```python
from build123d import *

# Parameters (mm, degrees)
BOSS_EXTRUDE1_START     = -21.43125
SKETCH4_R               = 6.35
BOSS_EXTRUDE1_DEPTH     = 42.8625
SKETCH5_R               = 1.984375
CUT_EXTRUDE1_DEPTH      = 42.828441001
CHAMFER1_SIZE           = 0.6985
CUT_EXTRUDE3_REACH      = 52.483
CUT_EXTRUDE3_END_RADIUS = 6.35
SKETCH7_R               = 2.4257


with BuildPart() as part:
    # Sketch4 → Boss-Extrude1 (new body)
    with BuildSketch(Plane.XY.offset(BOSS_EXTRUDE1_START)):
        with BuildLine():
            Line((-25.4, -9.525), (-17.4625, -9.525))
            Line((-17.4625, -9.525), (-17.4625, 12.7))
            Line((-17.4625, 12.7), (-10.4775, 12.7))
            ThreePointArc((-10.4775, 12.7), (0, 15.875), (10.4775, 12.7))
            Line((10.4775, 12.7), (17.4625, 12.7))
            Line((17.4625, 12.7), (17.4625, -9.525))
            Line((17.4625, -9.525), (25.4, -9.525))
            Line((25.4, -9.525), (25.4, -15.875))
            Line((25.4, -15.875), (9.42975, -15.875))
            Line((9.42975, -15.875), (9.42975, -15.5575))
            Line((9.42975, -15.5575), (-9.42975, -15.5575))
            Line((-9.42975, -15.5575), (-9.42975, -15.875))
            Line((-9.42975, -15.875), (-25.4, -15.875))
            Line((-25.4, -15.875), (-25.4, -9.525))
        make_face()
        with Locations((0, 1.5748)):
            Circle(SKETCH4_R, mode=Mode.SUBTRACT)
    extrude(amount=BOSS_EXTRUDE1_DEPTH)

    # Sketch5 → Cut-Extrude1 (cut, through all)
    with BuildSketch(Plane(origin=(0, -9.525, 0), x_dir=(1, 0, 0), z_dir=(0, 1, 0))):
        with Locations(Location((-21.4376, 12.7, 0), (0, 0, 180))):
            Circle(SKETCH5_R)
        with Locations(Location((21.4376, 12.7, 0), (0, 0, 180))):
            Circle(SKETCH5_R)
        with Locations(Location((21.4376, -12.7, 0), (0, 0, 180))):
            Circle(SKETCH5_R)
        with Locations(Location((-21.4376, -12.7, 0), (0, 0, 180))):
            Circle(SKETCH5_R)
    extrude(amount=-CUT_EXTRUDE1_DEPTH, mode=Mode.SUBTRACT)

    # Chamfer1
    chamfer1_edges = [part.edges().sort_by_distance(p)[0] for p in [
        (-17.4625, 12.7, 0),
        (17.4625, 12.7, 0),
    ]]
    chamfer(chamfer1_edges, length=CHAMFER1_SIZE)

    # Cut-Extrude3: up to this cylinder (the profile starts outside it)
    cut_extrude3_end = Plane(origin=(0, 1.5748, 0), z_dir=(0, 0, -1)) * Cylinder(CUT_EXTRUDE3_END_RADIUS, 118.666, mode=Mode.PRIVATE)
    # Sketch7 → Cut-Extrude3 (cut, up to the surface)
    with BuildSketch(Plane(origin=(17.4625, 0, 0), x_dir=(0, 0, -1), z_dir=(1, 0, 0)), mode=Mode.PRIVATE) as cut_extrude3_sk1:
        with Locations((0, 1.5748)):
            Circle(SKETCH7_R)
    cut_extrude3_tool1 = extrude(cut_extrude3_sk1.sketch, amount=-CUT_EXTRUDE3_REACH, mode=Mode.PRIVATE) - cut_extrude3_end
    add(cut_extrude3_tool1.solids().sort_by_distance((17.4625, 1.5748, 0))[0], mode=Mode.SUBTRACT)


solid = part.part
```
Here's how the part is built. I have some questions about the finished solid (model axes, mm). A direction names the side the tool comes from. Give positions to 0.01 mm unless a question says otherwise; leave off trailing zeros. Loops run counter-clockwise (first coordinate to the right, second up) from the corner with the lowest first, then second, coordinate; pieces in that order, holes last. Notation, with made-up numbers: (-20, -37.75) -> (37, -37.75) arc R27 cw to (37, -5.75) -> close; hole circle Ø1 at (43, -36.5). An arc over 180 degrees is marked (long way). Use one line per item in the form item = value. Start each with the question number.
1) Which directions (+Z, -Z, +X, -X, +Y, -Y) give clear straight access to the entire face, cutting with the end or side of a thin tool? Please do faces 4 (the face through (-17, -15.875, 0)), 5 (the face through (-14, 12.7, 0)), 6 (the face through (11.746, -0.577, -1.119)), 7 (the face through (25.4, -13, 0)), 8 (the face through (17.462, -1, -0.3)).
2) Imagine slicing it at B-B (y = -13). Please give me the cut outline in (x, z).
3) Imagine slicing it at A-A (x = 0). Please give me the cut outline in (y, z) (1 decimal).
4) Imagine slicing it at D-D (y = 7). Please give me the cut outline in (x, z).
5) Thinking about a two-plate mould opening in X: for faces 1 (the face through (0, -15.558, 0)), 2 (the face through (0, -7, -21.431)), 3 (the face through (-17.462, 1, 0)), which applies, +X half, -X half, draft (parallel to the pull), parting line (faces both ways), or undercut?
6) Imagine slicing it at C-C (z = 12.7). Count the separate pieces of the cut face and the enclosed holes in it, then the cut area to 3 significant figures.
7) For P1, Ø1, axis at x = -2, z = 5.5, coming from the +Y side; P2, Ø3, axis at x = -21.44, z = -12.7, coming from the +Y side; P3, Ø6.5, axis at y = 4.5, z = 3, coming from the -X side; P4, Ø5, axis at y = 3.5, z = -5, coming from the +X side, each with a flat end and sliding along its axis, tell me the tip position at first contact or that it passes through.
8) Please list where these lines run through material, in increasing order: line 1 along Y through (x, z) = (0, 3) (1 decimal); line 2 along X through (y, z) = (-12, -12); line 3 along Y through (x, z) = (11, 0) (1 decimal).
Check values:
q1.face_4 = +Z, -Z, +X, -X, -Y
q1.face_5 = +Z, -Z, -X, +Y
q1.face_6 = +X
q1.face_7 = +Z, -Z, +X, +Y, -Y
q1.face_8 = +Z, -Z, +X, +Y
q2.outline = (-25.4, -21.43) -> (25.4, -21.43) -> (25.4, 21.43) -> (-25.4, 21.43) -> close; hole circle Ø3.97 at (-21.44, -12.7); hole circle Ø3.97 at (-21.44, 12.7); hole circle Ø3.97 at (21.44, -12.7); hole circle Ø3.97 at (21.44, 12.7)
q3.outline = (-15.6, -21.4) -> (-4.8, -21.4) -> (-4.8, 21.4) -> (-15.6, 21.4) -> close; (7.9, -21.4) -> (15.9, -21.4) -> (15.9, 21.4) -> (7.9, 21.4) -> close
q4.outline = (-17.46, -21.43) -> (-3.3, -21.43) -> (-3.3, 21.43) -> (-17.46, 21.43) -> close; (3.3, -21.43) -> (17.46, -21.43) -> (17.46, 21.43) -> (3.3, 21.43) -> close
q5.face_1 = undercut
q5.face_2 = draft
q5.face_3 = -X half
q6.separate_pieces = 3
q6.enclosed_holes = 1
q6.area = 960 mm^2
q7.P1 = 15.82
q7.P2 = through
q7.P3 = -17.46
q7.P4 = 17.46
q8.line_1 = -15.6 to -4.8, 7.9 to 15.9
q8.line_2 = -25.4 to -23.29, -19.58 to 19.58, 23.29 to 25.4
q8.line_3 = -15.9 to -0.9, 4 to 12.7
